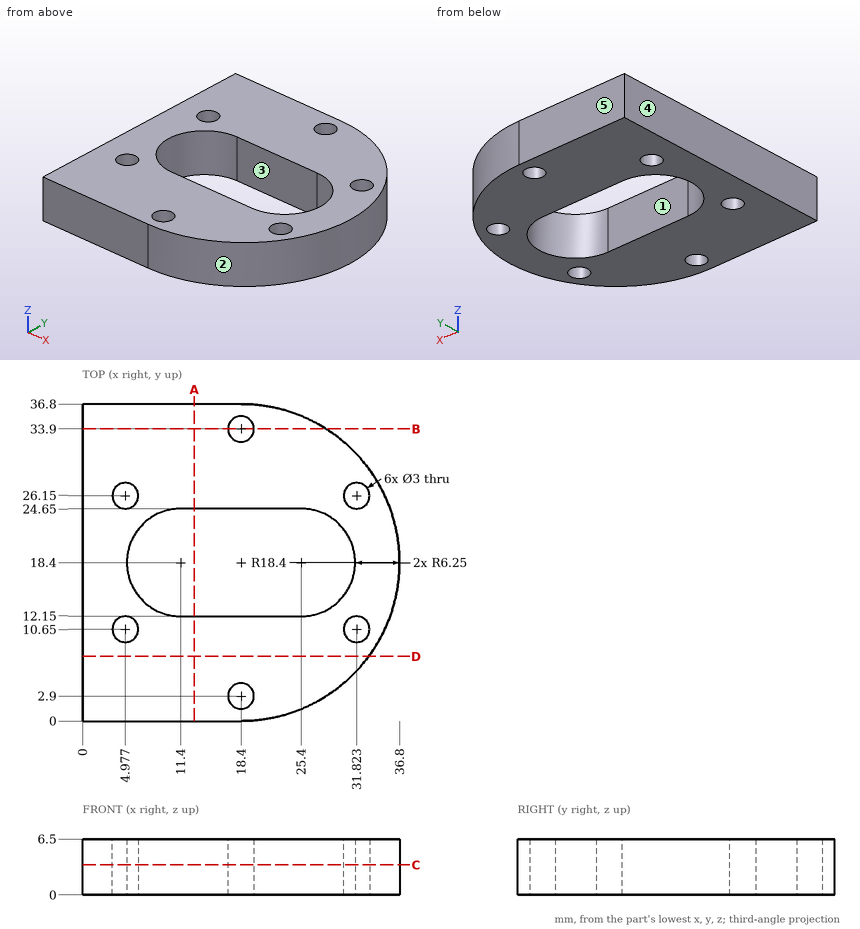
Here's the drawing with two shaded views (mm, measured from the low corner). I have some questions. A direction names the side the tool comes from. Coordinates: 2 decimals unless noted, no trailing zeros. Write each loop counter-clockwise with the first axis right and the second up, starting at its lowest first coordinate (ties: lowest second). Pieces come first, ordered by that corner, then holes.
Item 1: I want a section at A-A on x = 13. Write out the boundary of the cut face in (y, z).
Item 2: On a 3-axis mill with a long thin cutter (end or side, diameter ignored), from which of +Z, -Z, +X, -X, +Y, -Y can I reach the whole of each face in a straight line? I mean the marked faces 1 and 2. Say none if no direction works.
Item 3: I want a section at B-B on y = 33.9. Write out the boundary of the cut face in (x, z) (1 decimal).
Item 4: If I drill on line 1 (Y direction, x = 18.5, z = 3); line 2 (Y direction, x = 26, z = 4); line 3 (Y direction, x = 4, z = 3.25), over which ranges is the centre line in solid material (lowest first)?
Item 5: I want a section at C-C on z = 3.5. Write out the boundary of the cut face in (x, y).
Item 6: I want a section at D-D on y = 7.5. Write out the boundary of the cut face in (x, z).
Item 7: Will these pins go through, and if not, where does the flat tip stop? pin 1 (3.5 mm diameter, centred on x = 31.82, y = 26.15, fed in from -Z); pin 2 (2.5 mm diameter, centred on x = 4.98, y = 10.65, fed in from -Z); pin 3 (2 mm diameter, centred on y = 14, z = 0.5, fed in from +X); pin 4 (3 mm diameter, centred on y = 5.5, z = 3, fed in from +X).
Item 8: If we mould it in two halves opening along X, with no side actions, what happens to the marked faces 3, 4 and 5? For each: +X half, -X half, draft (parallel to the pull), parting line (faces both ways), or undercut.
Findings below:
1. outline: (0, 0) - (12.15, 0) - (12.15, 6.5) - (0, 6.5) - close; (24.65, 0) - (36.8, 0) - (36.8, 6.5) - (24.65, 6.5) - close
2. face 1: +Z, -Z
2. face 2: +Z, -Z, +X
3. outline: (0, 0) - (16.9, 0) - (16.9, 6.5) - (0, 6.5) - close; (19.9, 0) - (28.3, 0) - (28.3, 6.5) - (19.9, 6.5) - close
4. line 1: y = 0 to 1.4, 4.4 to 12.15, 24.65 to 32.4, 35.4 to 36.8
4. line 2: y = 1.64 to 12.18, 24.62 to 35.16
4. line 3: y = 0 to 9.51, 11.79 to 25.01, 27.29 to 36.8
5. outline: (0, 0) - (18.4, 0) arc R18.4 ccw to (18.4, 36.8) - (0, 36.8) - close; hole circle Ø3 at (4.98, 10.65); hole circle Ø3 at (4.98, 26.15); hole (11.4, 12.15) - (25.4, 12.15) arc R6.25 ccw to (25.4, 24.65) - (11.4, 24.65) arc R6.25 ccw to start; hole circle Ø3 at (18.4, 2.9); hole circle Ø3 at (18.4, 33.9); hole circle Ø3 at (31.82, 10.65); hole circle Ø3 at (31.82, 26.15)
6. outline: (0, 0) - (33.22, 0) - (33.22, 6.5) - (0, 6.5) - close
7. pin 1: stops at z = 0
7. pin 2: passes through
7. pin 3: stops at x = 36.48
7. pin 4: stops at x = 32.84
8. face 3: undercut
8. face 4: -X half
8. face 5: draft
